The listing builds one solid part. Answer for the finished solid, in the listing's coordinates (mm). Face numbers are marked on the shaded views. A direction names the side the tool comes from. Coordinates: 2 decimals unless noted, no trailing zeros. Loops run counter-clockwise (first coordinate to the right, second up) from the corner with the lowest first, then second, coordinate; pieces in that order, holes last. Notation, with made-up numbers: M -15,9 L 18,9 A10 ccw 18,13 Z; hole C 42.5,-35.5 d3. An arc over 180 degrees is marked long. Answer as CSV lines item,"result". Start each with the question number.
```python
from build123d import *

# Parameters (mm, degrees)
CROQUIS1_R              = 6
SALIENTE_EXTRUIR1_DEPTH = 2.5
CROQUIS2_R              = 6
SALIENTE_EXTRUIR2_DEPTH = 5.5
CROQUIS3_R              = 1.5
CORTAR_EXTRUIR1_DEPTH   = 12.5
CROQUIS4_R              = 3
CORTAR_EXTRUIR2_DEPTH   = 3
CROQUIS5_R              = 9
CROQUIS5_R_2            = 3
SALIENTE_EXTRUIR3_DEPTH = 3
REDONDEO1_R             = 2


with BuildPart() as part:
    # Croquis1 → Saliente-Extruir1 (new body)
    with BuildSketch(Plane.ZY.offset(24.669607513)):
        with Locations((65.25, -8.936333162)):
            Circle(CROQUIS1_R)
        Polygon((67.674871131, -4.736333162), (62.825128869, -4.736333162), (60.400257739, -8.936333162), (62.825128869, -13.136333162), (67.674871131, -13.136333162), (70.099742261, -8.936333162), align=None, mode=Mode.SUBTRACT)
    extrude(amount=SALIENTE_EXTRUIR1_DEPTH)

    # Croquis2 → Saliente-Extruir2 (add)
    with BuildSketch(Plane.ZY.offset(27.169607513)):
        with Locations((65.25, -8.936333162)):
            Circle(CROQUIS2_R)
    extrude(amount=SALIENTE_EXTRUIR2_DEPTH)

    # Croquis3 → Cortar-Extruir1 (cut)
    with BuildSketch(Plane.ZY.offset(32.669607513)):
        with Locations((65.25, -8.936333162)):
            Circle(CROQUIS3_R)
    extrude(amount=-CORTAR_EXTRUIR1_DEPTH, mode=Mode.SUBTRACT)

    # Croquis4 → Cortar-Extruir2 (cut)
    with BuildSketch(Plane.ZY.offset(32.669607513)):
        with Locations((65.25, -8.936333162)):
            Circle(CROQUIS4_R)
    extrude(amount=-CORTAR_EXTRUIR2_DEPTH, mode=Mode.SUBTRACT)

    # Croquis5 → Saliente-Extruir3 (add)
    with BuildSketch(Plane.ZY.offset(31.069607513)):
        with Locations((65.25, -8.936333162)):
            Circle(CROQUIS5_R)
        with Locations((65.25, -8.936333162)):
            Circle(CROQUIS5_R_2, mode=Mode.SUBTRACT)
    extrude(amount=SALIENTE_EXTRUIR3_DEPTH)

    # Redondeo1
    redondeo1_edges = [part.edges().sort_by_distance(p)[0] for p in [
        (-34.069607513, -8.936333162, 56.25),
    ]]
    fillet(redondeo1_edges, radius=REDONDEO1_R)


solid = part.part
```
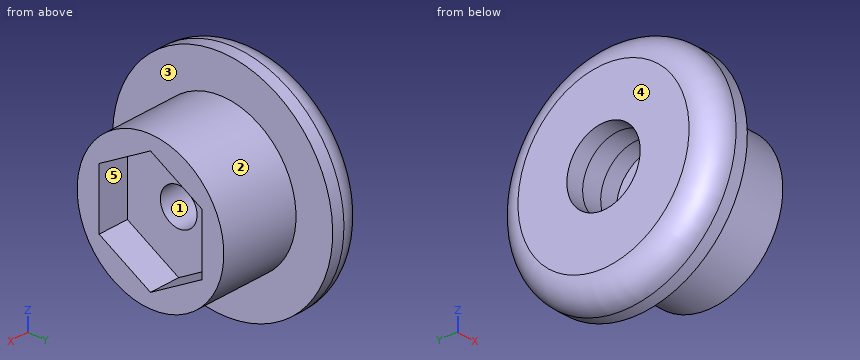
Item 1: For the marked faces 4 and 5, determine the directions among +Z, -Z, +X, -X, +Y, -Y from which every point of the face is accessible in a straight line to the end or side of a thin tool.
Item 2: Section B-B on x = -25.5 is taken. Determine the outline of the cut face in (y, z), then the cut area to 3 significant figures.
Item 3: Consider line 1 (Y direction, x = -32.1, z = 65.25); line 2 (Y direction, x = -29.75, z = 66.5); line 3 (X direction, y = -14.25, z = 69.5). Determine where each line is inside the solid, lowest interval first.
Item 4: Section D-D on x = -29 is taken. Determine the outline of the cut face in (y, z).
Item 5: For a pull along Z with two mould halves and no side action, classify the marked faces 1, 2 and 3 as pulls with the +Z half, pulls with the -Z half, needs draft (parallel to the pull), parting line crosses it, or undercut.
Item 6: Each of these flat-tipped pins is pushed along its axis until it touches: P1, Ø4, axis at y = -8, z = 67, coming from the +X side; P2, Ø0.8, axis at x = -25.5, z = 64.5, coming from the +Y side; P3, Ø1, axis at y = -15, z = 58.5, coming from the -X side; P4, Ø1.8, axis at y = -8.94, z = 65.25, coming from the -X side. Where does it stop, or does it pass through?
Item 7: Section C-C on x = -30.75 is taken. Determine the outline of the cut face in (y, z), then the cut area to 3 significant figures.
Item 8: Section A-A on z = 65.25 is taken. Determine the outline of the cut face in (x, y), then the cut area to 3 significant figures.
Results are:
1,face 4,"+Z, -Z, -X, +Y, -Y"
1,face 5,"+X"
2,outline,"C -8.94,65.25 d12; hole M -13.14,62.83 L -8.94,60.4 L -4.74,62.83 L -4.74,67.67 L -8.94,70.1 L -13.14,67.67 Z"
2,area,"52.0 mm²"
3,line 1,"-17.94 to -11.94, -5.94 to 0.06"
3,line 2,"-14.8 to -11.66, -6.21 to -3.07"
3,line 3,"-34.07 to -31.07"
4,outline,"C -8.94,65.25 d12; hole C -8.94,65.25 d3"
5,face 1,"undercut"
5,face 2,"parting line crosses it"
5,face 3,"needs draft"
6,P1,"x = -27.17"
6,P2,"y = -2.95"
6,P3,"x = -33.3"
6,P4,"through"
7,outline,"C -8.94,65.25 d12; hole C -8.94,65.25 d6"
7,area,"84.8 mm²"
8,outline,"M -34.07,-15.94 A2 ccw -32.07,-17.94 L -31.07,-17.94 L -31.07,-14.94 L -24.67,-14.94 L -24.67,-13.14 L -27.17,-13.14 L -27.17,-10.44 L -29.67,-10.44 L -29.67,-11.94 L -34.07,-11.94 Z; M -34.07,-5.94 L -29.67,-5.94 L -29.67,-7.44 L -27.17,-7.44 L -27.17,-4.74 L -24.67,-4.74 L -24.67,-2.94 L -31.07,-2.94 L -31.07,0.06 L -32.07,0.06 A2 ccw -34.07,-1.94 Z"
8,area,"74.2 mm²"
